from build123d import *

# Parameters (mm, degrees)
F0_W      = 19.05
F0_H      = 19.05
F1_DEPTH  = 12.7
F2_R      = 3.96875
F3_DEPTH  = 12.701
F10_DEPTH = 12.7


with BuildPart() as f1:
    # F0 (on Top) → F1 (new body)
    with BuildSketch(Plane.XY):
        Rectangle(F0_W, F0_H)
    extrude(amount=F1_DEPTH)

    # F2 (on face) → F3 (cut, through all)
    with BuildSketch(Plane.XY.offset(12.7)):
        Circle(F2_R)
    extrude(amount=-F3_DEPTH, mode=Mode.SUBTRACT)

    # F4 (on Right) → F5 (revolve, cut)
    with BuildSketch(Plane.YZ):
        Polygon((24.765, 12.7), (9.525, 12.7), (24.765, 8.6164543073), align=None)
    revolve(axis=Axis((0, 0, 12.7), (0, 0, 1)), mode=Mode.SUBTRACT)

    # F7 (on Right) → F8 (revolve, cut)
    with BuildSketch(Plane.YZ):
        Polygon((-22.8305501432, 0), (-9.525, 0), (-22.8305501432, 3.5652114157), align=None)
    revolve(axis=Axis((0, 0, 0), (0, 0, -1)), mode=Mode.SUBTRACT)

    # F9 (on Front) → F10 (cut, symmetric)
    with BuildSketch(Plane.XZ):
        Polygon((-8.7912914261, 6.35), (-9.525, 6.35), (-9.525, 5.6162914261), align=None)
        Polygon((-8.7912914261, 6.35), (-9.525, 7.0837085739), (-9.525, 6.35), align=None)
    extrude(amount=F10_DEPTH, both=True, mode=Mode.SUBTRACT)


solid = f1.part
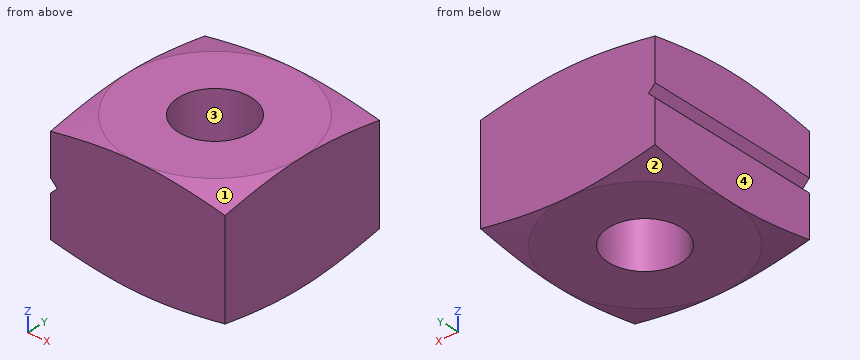
The listing builds one solid part. Answer for the finished solid, in the listing's coordinates (mm). Face numbers are marked on the shaded views. Coordinates: 2 decimals unless noted, no trailing zeros. Loops run counter-clockwise (first coordinate to the right, second up) from the corner with the lowest first, then second, coordinate; pieces in that order, holes last. Notation, with made-up numbers: M -33.5,-24 L 4.5,-24 A24 cw 4.5,-10 Z; hole C 24.25,38.5 d6. An arc over 180 degrees is marked long. Answer in a Markdown table with one row per item.
1) Find the intervals of material crossed by probe 1 along Y at (x, z) = (0, 6.5) (3 decimals); probe 2 along Y at (x, z) = (-3.25, 5) (3 decimals); probe 3 along X at (y, z) = (1.75, 6.75) (3 decimals), in increasing order.
Answers below:
| item | result |
|---|---|
| probe 1 | -9.525 to -3.969, 3.969 to 9.525 |
| probe 2 | -9.525 to -2.278, 2.278 to 9.525 |
| probe 3 | -9.191 to -3.562, 3.562 to 9.525 |
2) Find section A-A (z = 3). Determine the outline of the cut face in (x, y) (1 decimal), then the cut area to 3 significant figures.
Answers below:
| item | result |
|---|---|
| outline | M -9.5,-9.5 L 9.5,-9.5 L 9.5,9.5 L -9.5,9.5 Z; hole C 0,0 d7.9 |
| area | 313 mm^2 |
3) Determine the mould class of the marked faces 1, 2, 3 and 4 for opening direction Y: released by +Y, released by -Y, zero draft, split by the parting line, or undercut.
Answers below:
| item | result |
|---|---|
| face 1 | released by -Y |
| face 2 | released by +Y |
| face 3 | undercut |
| face 4 | zero draft |
4) Given pin 1 (5 mm diameter, centred on x = 0, y = 0, fed in from -Z), flat-ended and moving along its own axis, determine where the tip first touches the part or whether it passes through.
Answers below:
| item | result |
|---|---|
| pin 1 | through |
